Autodesk Inventor part; units mm, degrees
ref_plane "YZ Plane" through (0, 0, 0) normal (1, 0, 0) x (0, 1, 0)
ref_plane "XZ Plane" through (0, 0, 0) normal (0, 1, 0) x (-1, 0, 0)
ref_plane "XY Plane" through (0, 0, 0) normal (0, 0, 1) x (1, 0, 0)
sketch "Sketch1" plane through (0, 0, 0) normal (0, 1, 0) x (-1, 0, 0)
  line L0 (0, 0) -> (127, 0)
  line L1 (127, 0) -> (127, -50.8)
  line L2 (127, -50.8) -> (0, -50.8)
  line L3 (0, -50.8) -> (0, 0)
  dimension "d0" = 127
  dimension "d1" = 50.8
extrude "Extrusion1" add sketch "Sketch1" along normal blind 6.35
sketch "Sketch2" plane through (0, 6.35, 0) normal (0, 1, 0) x (1, 0, 0)
  circle A0 centre (-99.441, 25.4) radius 14.2875
  line L0 (0, 0) -> (0, 50.8)
  dimension "d4" = 28.575
  dimension "d5" = 99.441
extrude "Extrusion2" cut sketch "Sketch2" against normal blind 6.35
sketch "Sketch3" plane through (0, 6.35, 0) normal (0, 1, 0) x (1, 0, 0)
  line L0 (0, 0) -> (0, 50.8)
  line L1 (0, 0) -> (-9.525, 11.8364)
  line L2 (0, 50.8) -> (-9.525, 38.9636)
  dimension "d8" = 27.1272
  dimension "d9" = 9.525
  dimension "d10" = 9.525
hole "Hole1" at (-9.525, 6.35, -11.8364) at (-9.525, 6.35, -38.9636) direction (0, -1, 0) diameter 6.5278 depth 25.4 tip angle 118
properties part number "Pin Support Plate"
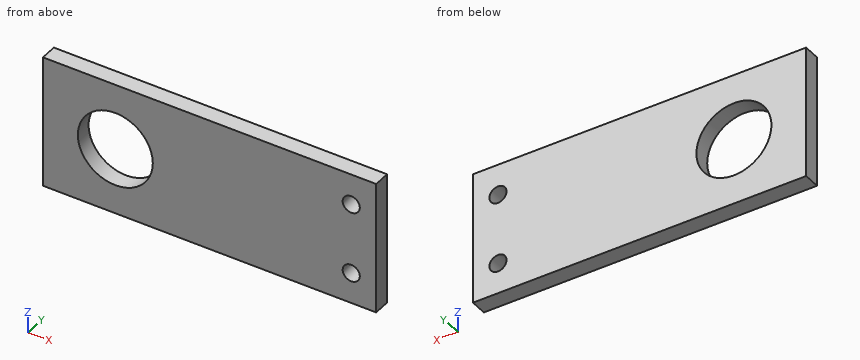
Input: part model. Units: mm. Frame: model coordinates. Round coordinates to 2 decimals unless told otherwise and drop trailing zeros. Loops run counter-clockwise (first coordinate to the right, second up) from the corner with the lowest first, then second, coordinate; pieces in that order, holes last.
1) Section query A-A on z = -25.4. Return the cut outline in (x, y).
Ans:
outline: (-127, 0) - (-113.73, 0) - (-113.73, 6.35) - (-127, 6.35) - close; (-85.15, 0) - (0, 0) - (0, 6.35) - (-85.15, 6.35) - close
2) Material intervals for line 1 (X direction, y = 6.25, z = -36); line 2 (X direction, y = 4, z = -25.4); line 3 (X direction, y = 5.5, z = -31), sorted ascending.
Ans:
line 1: x = -127 to -109.02, -89.86 to -10.89, -8.16 to 0
line 2: x = -127 to -113.73, -85.15 to 0
line 3: x = -127 to -112.59, -86.3 to 0
3) Section query C-C on x = -99.5. Return the cut outline in (y, z), plus the area to 3 significant figures.
Ans:
outline: (0, -50.8) - (6.35, -50.8) - (6.35, -39.69) - (0, -39.69) - close; (0, -11.11) - (6.35, -11.11) - (6.35, 0) - (0, 0) - close
area: 141 mm2
4) Section query B-B on y = 5.25. Return the cut outline in (x, z) (1 decimal), plus the area to 3 significant figures.
Ans:
outline: (-127, -50.8) - (0, -50.8) - (0, 0) - (-127, 0) - close; hole circle Ø28.6 at (-99.4, -25.4); hole circle Ø6.5 at (-9.5, -39); hole circle Ø6.5 at (-9.5, -11.8)
area: 5,740 mm2
5) Section query D-D on z = -14. Return the cut outline in (x, y).
Ans:
outline: (-127, 0) - (-108.05, 0) - (-108.05, 6.35) - (-127, 6.35) - close; (-90.83, 0) - (-11.97, 0) - (-11.97, 6.35) - (-90.83, 6.35) - close; (-7.08, 0) - (0, 0) - (0, 6.35) - (-7.08, 6.35) - close
